from build123d import *

# Parameters (mm, degrees)
SKETCH1_R           = 3.175
BOSS_EXTRUDE1_DEPTH = 38.1


with BuildPart() as part:
    # Sketch1 → Boss-Extrude1 (new body)
    with BuildSketch(Plane.XY):
        Polygon((-16.056683457, 2.733236781), (100.225653504, 2.733236781), (107.63663241, 88.047008638), (75.491893593, 61.490379753), (75.491893593, 20.88695082), (-16.056683457, 20.88695082), align=None)
        with Locations(Location((-8.634202411, 9.412425764, 0), (0, 0, 180))):
            Circle(SKETCH1_R, mode=Mode.SUBTRACT)
        with Locations(Location((92.965797589, 9.412425764, 0), (0, 0, 180))):
            Circle(SKETCH1_R, mode=Mode.SUBTRACT)
    extrude(amount=BOSS_EXTRUDE1_DEPTH)


solid = part.part
Work out the finished part from the listing and answer in its coordinate system (mm). A direction names the side the tool comes from. Round coordinates to 2 decimals unless told otherwise and drop trailing zeros. Order: outer loops, then holes, each group sorted by start corner. A loop starts at its lowest first (then second) coordinate and runs counter-clockwise, first axis right, second up. Notation, with made-up numbers: M 83.25,34.5 L 122.25,34.5 A17 ccw 122.25,67.5 Z; hole C 55,42 d7. An arc over 180 degrees is marked long. One line per item, written item: value.
Q1. Find section B-B on y = 83. Write down the section's boundary in (x, z).
Derived:
outline: M 101.53,0 L 107.2,0 L 107.2,38.1 L 101.53,38.1 Z
Q2. Find section C-C on x = 87. Write down the section's boundary in (y, z), then the cut area to 3 significant figures.
Derived:
outline: M 2.73,0 L 71,0 L 71,38.1 L 2.73,38.1 Z
area: 2,600 mm²
Q3. Straight lines are drawn through the part: line 1 (Y direction, x = 10, z = 13); line 2 (Y direction, x = -9, z = 5); line 3 (Y direction, x = -9.5, z = 14). For each, find the intervals that lie inside material, in ascending order.
Derived:
line 1: 2.73 to 20.89
line 2: 2.73 to 6.26, 12.57 to 20.89
line 3: 2.73 to 6.36, 12.47 to 20.89
Q4. Flat-ended cylindrical pins translate along their axes: pin 1 (11.5 mm diameter, centred on x = 47.5, z = 14.5, fed in from +Y); pin 2 (19 mm diameter, centred on y = 47.5, z = 27.5, fed in from -X); pin 3 (5 mm diameter, centred on x = 92.97, y = 9.41, fed in from -Z); pin 4 (6 mm diameter, centred on y = 20, z = 11.5, fed in from +X). Find the tip coordinate at first contact, or state that the pin passes through.
Derived:
pin 1: y = 20.89
pin 2: x = 75.49
pin 3: through
pin 4: x = 101.99
Q5. For faces 1 (the face through (64, 20, 0)), 2 (the face through (75.492, 41, 19)), determine the directions among +Z, -Z, +X, -X, +Y, -Y from which every point of the face is accessible in a straight line to the end or side of a thin tool.
Derived:
face 1: -Z, +X, -X, +Y, -Y
face 2: +Z, -Z, -X, +Y
Q6. Find section A-A on z = 18.5. Write down the section's boundary in (x, y) (3 decimals).
Derived:
outline: M -16.057,2.733 L 100.226,2.733 L 107.637,88.047 L 75.492,61.49 L 75.492,20.887 L -16.057,20.887 Z; hole C -8.634,9.412 d6.35; hole C 92.966,9.412 d6.35
Q7. Determine the mould class of faces 3 (the face through (91.789, 74.955, 18.783)), 4 (the face through (103.88, 44.79, 18.78)), 5 (the face through (41, 2.733, 19)), 6 (the face through (-5.462, 9.273, 18.783)) for opening direction X: released by +X, released by -X, zero draft, split by the parting line, or undercut.
Derived:
face 3: released by -X
face 4: released by +X
face 5: zero draft
face 6: undercut
